CAD build for the part. Positions are in the model's coordinates, mm. Round coordinates to 2 decimals unless told otherwise and drop trailing zeros. Loops run counter-clockwise (first coordinate to the right, second up) from the corner with the lowest first, then second, coordinate; pieces in that order, holes last.
from build123d import *

# Parameters (mm, degrees)
SKETCH4_R          = 1
SKETCH4_R_2        = 1.25
EXTRUDE2_DEPTH     = 8.8
SKETCH5_R          = 5
CUT_EXTRUDE1_DEPTH = 8.8


with BuildPart() as part:
    # Sketch1 → Revolve1 (revolve)
    with BuildSketch(Plane.XY):
        Polygon((6.609375, 15), (1.190625, 15), (0, 15), (0, 14), (0, 0), (7.8, 0), (7.8, 14), (7.8, 15), align=None)
    revolve(axis=Axis((0, 0, 0), (1, 0, 0)))

    # Sketch4 → Extrude2 (cut, through all)
    with BuildSketch(Plane(origin=(7.8, 0, 0), x_dir=(0, 0, -1), z_dir=(1, 0, 0))):
        with Locations((0, 11)):
            Circle(SKETCH4_R)
        with Locations((-4.381841494, 10.089572098)):
            Circle(SKETCH4_R_2)
        with Locations((4.381841494, 10.089572098)):
            Circle(SKETCH4_R_2)
        with Locations((10.089572098, -4.381841494)):
            Circle(SKETCH4_R_2)
        with Locations((11, 0)):
            Circle(SKETCH4_R)
        with Locations((10.089572098, 4.381841494)):
            Circle(SKETCH4_R_2)
        with Locations((-4.381841494, -10.089572098)):
            Circle(SKETCH4_R_2)
        with Locations((0, -11)):
            Circle(SKETCH4_R)
        with Locations((4.381841494, -10.089572098)):
            Circle(SKETCH4_R_2)
        with Locations((-10.089572098, 4.381841494)):
            Circle(SKETCH4_R_2)
        with Locations((-11, 0)):
            Circle(SKETCH4_R)
        with Locations((-10.089572098, -4.381841494)):
            Circle(SKETCH4_R_2)
    extrude(amount=-EXTRUDE2_DEPTH, mode=Mode.SUBTRACT)

    # Sketch5 → Cut-Extrude1 (cut, through all)
    with BuildSketch(Plane(origin=(7.8, 0, 0), x_dir=(0, 0, -1), z_dir=(1, 0, 0))):
        Circle(SKETCH5_R)
    extrude(amount=-CUT_EXTRUDE1_DEPTH, mode=Mode.SUBTRACT)


solid = part.part
Item 1: Cut at C-C (z = 9.25). List the corners of the cut face in (x, y), plus the area to 3 significant figures.
Verdict:
outline: (0, -11.81) - (7.8, -11.81) - (7.8, -5.31) - (0, -5.31) - close; (0, -3.46) - (7.8, -3.46) - (7.8, 3.46) - (0, 3.46) - close; (0, 5.31) - (7.8, 5.31) - (7.8, 11.81) - (0, 11.81) - close
area: 155 mm2
Item 2: Flat gauge pins, fed straight in: P1, Ø2, axis at y = -10.09, z = -4.38, coming from the +X side; P2, Ø3, axis at x = 2.5, y = -11.5, coming from the -Z side; P3, Ø1, axis at x = 7, z = 9.5, coming from the +Y side; P4, Ø1.5, axis at x = 2.5, z = -8.5, coming from the -Y side. Where does each tip first touch, or does it go through?
Verdict:
P1: passes through
P2: stops at z = -11.18
P3: stops at y = 12
P4: stops at y = -12.84
Item 3: Mould opens along Y. For faces 1 (the flat face through (0, -4, 4)), 2 (the cylindrical face through (4, 10, 0)), 3 (the cylindrical face through (3.845, -14.985, 0.66)) say: released by +Y, released by -Y, zero draft, split by the parting line, or undercut.
Verdict:
face 1: zero draft
face 2: undercut
face 3: split by the parting line
Item 4: Cut at A-A (z = 0). List the corners of the cut face in (x, y), plus the area to 3 significant figures.
Verdict:
outline: (0, -15) - (7.8, -15) - (7.8, -12) - (0, -12) - close; (0, -10) - (7.8, -10) - (7.8, -5) - (0, -5) - close; (0, 5) - (7.8, 5) - (7.8, 10) - (0, 10) - close; (0, 12) - (7.8, 12) - (7.8, 15) - (0, 15) - close
area: 125 mm2
Item 5: Wall check: L1, parallel to Z at x = 1.5, y = -4; L2, parallel to Z at x = 1.25, y = -9.75; L3, parallel to Z at x = 1.5, y = 10.25. Give the ranges that are in metal, low to high.
Verdict:
L1: z = -14.46 to -11.28, -8.9 to -3, 3 to 8.9, 11.28 to 14.46
L2: z = -11.4 to -5.58, -3.18 to 3.18, 5.58 to 11.4
L3: z = -10.95 to -5.62, -3.14 to -0.66, 0.66 to 3.14, 5.62 to 10.95
Item 6: Cut at D-D (x = 0.75). State how many separate pieces and enclosed holes the cut face has, plus the area to 3 significant figures.
Verdict:
separate pieces: 1
enclosed holes: 13
area: 576 mm2
